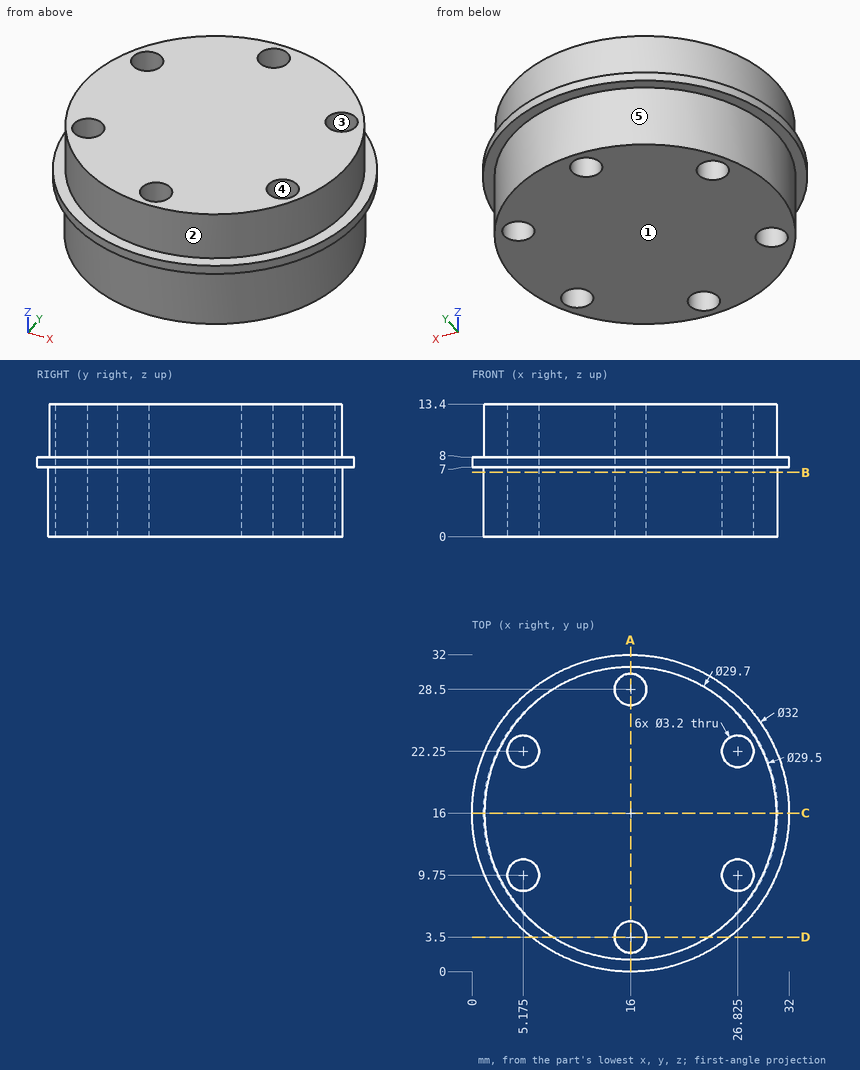
Verification items for this drawing (mm, ordinates from the low corner). A direction names the side the tool comes from. Coordinates: 2 decimals unless noted, no trailing zeros. Order: outer loops, then holes, each group sorted by start corner. A loop starts at its lowest first (then second) coordinate and runs counter-clockwise, first axis right, second up. Notation, with made-up numbers: (12, -18.5) - (29, -18.5) arc R27 cw to (29, 3.5) - close; hole circle Ø1 at (5, -12.5). An arc over 180 degrees is marked (long way). Answer as a JSON object with one key per item and string values. Group by question number.
Item 1: Draft check along X on the marked faces 1, 2 and 3. Enter one of: +X half, -X half, draft (parallel to the pull), parting line (faces both ways), or undercut.
Item 2: Sectioned sample at C-C, the plane y = 16. Record the cut outline in (x, z).
Item 3: Sectioned sample at A-A, the plane x = 16. Record the cut outline in (y, z).
Item 4: Depth check by flat-ended pin: pin 1 Ø1.5 at (x, z) = (22.5, 10) entering from +Y; pin 2 Ø1.9 at (x, y) = (26.83, 22.25) entering from -Z; pin 3 Ø4 at (x, y) = (8.5, 6) entering from -Z; pin 4 Ø3 at (x, z) = (25, 2.5) entering from -Y. Enter the tip coordinate at first touch or a pass-through.
Item 5: Tool access check on the marked faces 4 and 5. Record the directions out of +Z, -Z, +X, -X, +Y, -Y that give a thin tool (end or side, any length) a straight path to the whole face; none if there is none.
Item 6: Sectioned sample at D-D, the plane y = 3.5. Record the cut outline in (x, z), and give its area (3 significant figures).
Item 7: Sectioned sample at B-B, the plane z = 6.5. Give the number of separate pieces and of enclosed holes in the cut face.
Item 8: Scan lines: probe 1 along Y at (x, z) = (16, 10.25); probe 2 along X at (y, z) = (9.75, 6.75) (1 decimal); probe 3 along X at (y, z) = (22, 2.5) (1 decimal). Record each from-to range of solid material in increasing order.
Resolved:
{
 "1": {"face 1": "draft", "face 2": "parting line", "face 3": "undercut"},
 "2": {"outline": "(0, 7) - (1.15, 7) - (1.15, 0) - (30.85, 0) - (30.85, 7) - (32, 7) - (32, 8) - (30.75, 8) - (30.75, 13.4) - (1.25, 13.4) - (1.25, 8) - (0, 8) - close"},
 "3": {"outline": "(0, 7) - (1.15, 7) - (1.15, 0) - (1.9, 0) - (1.9, 13.4) - (1.25, 13.4) - (1.25, 8) - (0, 8) - close; (5.1, 0) - (26.9, 0) - (26.9, 13.4) - (5.1, 13.4) - close; (30.1, 0) - (30.85, 0) - (30.85, 7) - (32, 7) - (32, 8) - (30.75, 8) - (30.75, 13.4) - (30.1, 13.4) - close"},
 "4": {"pin 1": "y = 29.58", "pin 2": "through", "pin 3": "z = 0", "pin 4": "y = 3.18"},
 "5": {"face 4": "+Z, -Z", "face 5": "-Z"},
 "6": {"outline": "(6.01, 7) - (7.98, 7) - (7.98, 0) - (14.4, 0) - (14.4, 13.4) - (8.17, 13.4) - (8.17, 8) - (6.01, 8) - close; (17.6, 0) - (24.02, 0) - (24.02, 7) - (25.99, 7) - (25.99, 8) - (23.83, 8) - (23.83, 13.4) - (17.6, 13.4) - close", "area": "174 mm^2"},
 "7": {"separate pieces": "1", "enclosed holes": "6"},
 "8": {"probe 1": "1.25 to 1.9, 5.1 to 26.9, 30.1 to 30.75", "probe 2": "2.5 to 3.6, 6.8 to 25.2, 28.4 to 29.5", "probe 3": "2.4 to 3.6, 6.8 to 25.2, 28.4 to 29.6"}
}
